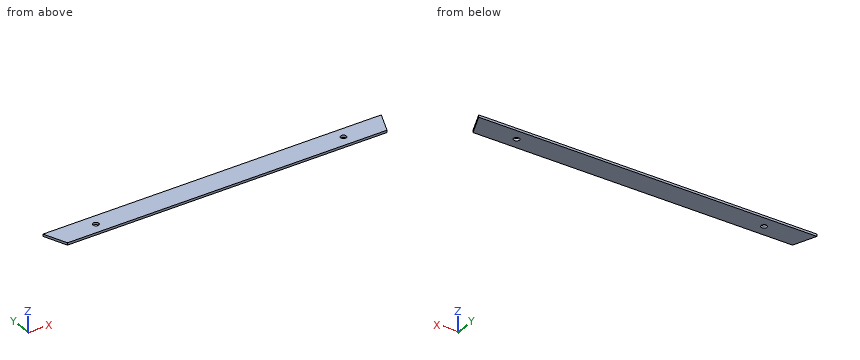
```python
from build123d import *

# Parameters (mm, degrees)
F0_W     = 378.7394
F0_H     = 25.4
F1_DEPTH = 2.54
F3_DEPTH = 2.541
F5_DEPTH = 2.541


with BuildPart() as f1:
    # F0 (on Top) → F1 (new body)
    with BuildSketch(Plane.XY):
        with Locations((42.002925, -34.459395)):
            Rectangle(F0_W, F0_H)
    extrude(amount=F1_DEPTH)

    # F2 (on face) → F3 (cut, through all)
    with BuildSketch(Plane.XY.offset(2.54)):
        Polygon((-136.846095, -47.159395), (-147.366775, -21.759395), (-147.366775, -47.159395), align=None)
        Polygon((231.372625, -47.159395), (231.372625, -21.759395), (220.851945, -47.159395), align=None)
    extrude(amount=-F3_DEPTH, mode=Mode.SUBTRACT)

    # F4 (on face) → F5 (cut, through all)
    with BuildSketch(Plane.XY.offset(2.54)):
        with BuildLine():
            ThreePointArc((-99.312349, -32.86489), (-97.392435, -37.52516), (-93.391775, -34.459395))
            ThreePointArc((-93.391775, -34.459395), (-95.741115, -31.393631), (-99.312349, -32.86489))
        make_face()
        with BuildLine():
            ThreePointArc((177.397625, -34.459395), (180.572625, -37.634395), (183.747625, -34.459395))
            ThreePointArc((183.747625, -34.459395), (180.572625, -31.284395), (177.397625, -34.459395))
        make_face()
    extrude(amount=-F5_DEPTH, mode=Mode.SUBTRACT)


solid = f1.part
```
The listing builds one solid part. Answer for the finished solid, in the listing's coordinates (mm). Coordinates: 2 decimals unless noted, no trailing zeros. Loops run counter-clockwise (first coordinate to the right, second up) from the corner with the lowest first, then second, coordinate; pieces in that order, holes last. Notation, with made-up numbers: (-35.5, -23.75) - (14.5, -23.75) arc R11 cw to (14.5, -9.75) - close; hole circle Ø2 at (25, -18.5). An arc over 180 degrees is marked (long way). Use a Markdown table: item, result. Add a question column.
1) Given pin 1 (5 mm diameter, centred on x = -96.57, y = -34.46, fed in from +Z), flat-ended and moving along its own axis, determine where the tip first touches the part or whether it passes through.
2) The part is cut by section B-B, the plane y = -43.75. Give the vertices of the cut face in (x, z), and give its area (3 significant figures).
3) The part is cut by section A-A, the plane z = 0.5. Give the vertices of the cut face in (x, y) (3 decimals).
4) Find the intervals of material crossed by line 1 (X direction, y = -35, z = 0.2); line 2 (X direction, y = -35.5, z = 1.8); line 3 (Y direction, x = 182, z = 1.7), in increasing order.
Here are the results:
| question | item | result |
|---|---|---|
| 1 | pin 1 | passes through |
| 2 | outline | (-138.26, 0) - (222.26, 0) - (222.26, 2.54) - (-138.26, 2.54) - close |
| 2 | area | 916 mm^2 |
| 3 | outline | (-147.367, -21.759) - (-136.846, -47.159) - (220.852, -47.159) - (231.373, -21.759) - close; hole circle Ø6.35 at (-96.567, -34.459); hole circle Ø6.35 at (180.573, -34.459) |
| 4 | line 1 | x = -141.88 to -99.7, -93.44 to 177.44, 183.7 to 225.89 |
| 4 | line 2 | x = -141.68 to -99.57, -93.57 to 177.57, 183.57 to 225.68 |
| 4 | line 3 | y = -47.16 to -37.3, -31.62 to -21.76 |
